Build history of the part. All positions in model axes, mm. Coordinates: 2 decimals unless noted, no trailing zeros. Order: outer loops, then holes, each group sorted by start corner. A loop starts at its lowest first (then second) coordinate and runs counter-clockwise, first axis right, second up. Notation, with made-up numbers: (82, -8.75) - (140, -8.75) arc R9 cw to (140, 8.25) - close; hole circle Ø4 at (80, 48.5). An arc over 180 degrees is marked (long way). Return JSON: item names as keys, results as strings.
from build123d import *

# Parameters (mm, degrees)
SKETCH1_R           = 2.25
BOSS_EXTRUDE2_DEPTH = 3.175


with BuildPart() as part:
    # Sketch1 → Boss-Extrude2 (new body)
    with BuildSketch(Plane(origin=(0, 0, 0), x_dir=(0, 0, -1), z_dir=(1, 0, 0))):
        Polygon((-70.039073078, -1.218967506), (59.322512202, -1.218967506), (99.611526043, -20.0060432), (99.611526043, -51.5060432), (83.611526043, -51.5060432), (83.611526043, -48.0060432), (47.611526043, -31.218967506), (-22.388473957, -31.218967506), (-41.758526434, -47.472371395), (-70.039073078, -47.472371395), align=None)
        with Locations((-57.538473957, -13.972371395)):
            Circle(SKETCH1_R, mode=Mode.SUBTRACT)
        with Locations((-57.538473957, -32.472371395)):
            Circle(SKETCH1_R, mode=Mode.SUBTRACT)
    extrude(amount=BOSS_EXTRUDE2_DEPTH)


solid = part.part
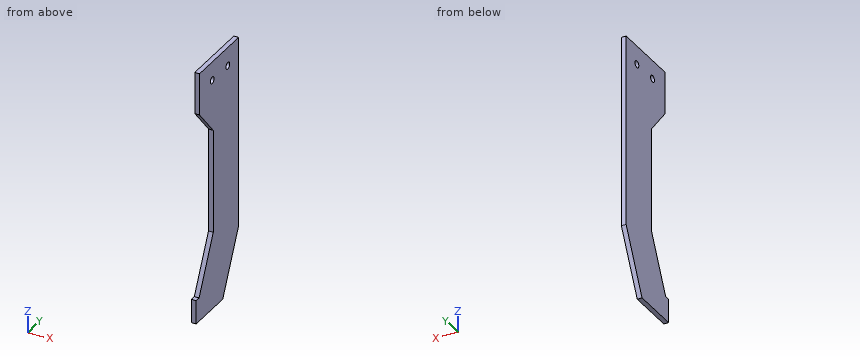
1. Cut at C-C on y = -5.5. Give the cut face in (x, z) (3 decimals).
Check values:
{"outline": "(0, -68.503) - (3.175, -68.503) - (3.175, 70.039) - (0, 70.039) - close"}
2. Cut at A-A on x = 1.15. Give the cut face in (y, z).
Check values:
{"outline": "(-51.51, -99.61) - (-20.01, -99.61) - (-1.22, -59.32) - (-1.22, 70.04) - (-47.47, 70.04) - (-47.47, 41.76) - (-31.22, 22.39) - (-31.22, -47.61) - (-48.01, -83.61) - (-51.51, -83.61) - close; hole circle Ø4.5 at (-32.47, 57.54); hole circle Ø4.5 at (-13.97, 57.54)"}
3. Probe L1, parallel to Z at x = 2.25, y = -31.5; L2, parallel to Z at x = 2.7, y = -32; L3, parallel to Y at x = 2.75, z = -5.5. List the from-to ranges inside material, lowest first.
Check values:
{"L1": "-99.61 to -48.21, 22.72 to 55.51, 59.57 to 70.04", "L2": "-99.61 to -49.29, 23.32 to 55.34, 59.74 to 70.04", "L3": "-31.22 to -1.22"}
4. Drop flat-ended pins along their axis: pin 1 (1.6 mm diameter, centred on x = 2.5, z = 55, fed in from -Y); pin 2 (1 mm diameter, centred on x = 2.5, y = -49.5, fed in from +Z); pin 3 (4 mm diameter, centred on y = -13.97, z = 57.54, fed in from +X); pin 4 (1.6 mm diameter, centred on x = 1, z = -4.5, fed in from -Y). Give the stop position or say it passes through.
Check values:
{"pin 1": "y = -47.47", "pin 2": "z = -83.61", "pin 3": "through", "pin 4": "y = -31.22"}
5. Cut at B-B on z = -12. Give the cut face in (x, y) (3 decimals).
Check values:
{"outline": "(0, -31.219) - (3.175, -31.219) - (3.175, -1.219) - (0, -1.219) - close"}
